Geometry check sheet. Reference: drawing and pictorial views, mm from the part's lowest x, y, z. A direction names the side the tool comes from. Round coordinates to 2 decimals unless told otherwise and drop trailing zeros. Order: outer loops, then holes, each group sorted by start corner. A loop starts at its lowest first (then second) coordinate and runs counter-clockwise, first axis right, second up. Notation, with made-up numbers: (86.25, 89.5) -> (131.25, 89.5) arc R23 cw to (131.25, 128.5) -> close; hole circle Ø10 at (26, 4.25). An arc over 180 degrees is marked (long way). Return JSON: item names as keys, results as strings. Group by question number.
1) Section check D-D on x = 63. Enter the section's corners in (y, z) (1 decimal), plus the area to 3 significant figures.
2) Section check A-A on z = 13. Enter the section's corners in (x, y) (1 decimal), plus the area to 3 significant figures.
3) Section check B-B on y = 1.5. Enter the section's corners in (x, z) (1 decimal).
4) Tool access check on the marked faces 1, 2 and 3. Record the directions out of +Z, -Z, +X, -X, +Y, -Y that give a thin tool (end or side, any length) a straight path to the whole face; none if there is none.
5) Section check C-C on z = 1.5. Enter the section's corners in (x, y) (1 decimal), plus the area to 3 significant figures.
6) Depth check by flat-ended pin: pin 1 (10 mm diameter, centred on x = 67, z = 17, fed in from -Y); pin 2 (2.5 mm diameter, centred on x = 79, y = 2.5, fed in from +Z); pin 3 (2 mm diameter, centred on x = 49.5, z = 3, fed in from +Y); pin 4 (0.8 mm diameter, centred on x = 30, y = 4, fed in from +Z). Enter the tip coordinate at first touch or a pass-through.
7) Scan lines: L1, parallel to X at y = 1, z = 6 (1 decimal); L2, parallel to Y at x = 51.5, z = 1; L3, parallel to X at y = 7.5, z = 17.75. Record each from-to range of solid material in increasing order.
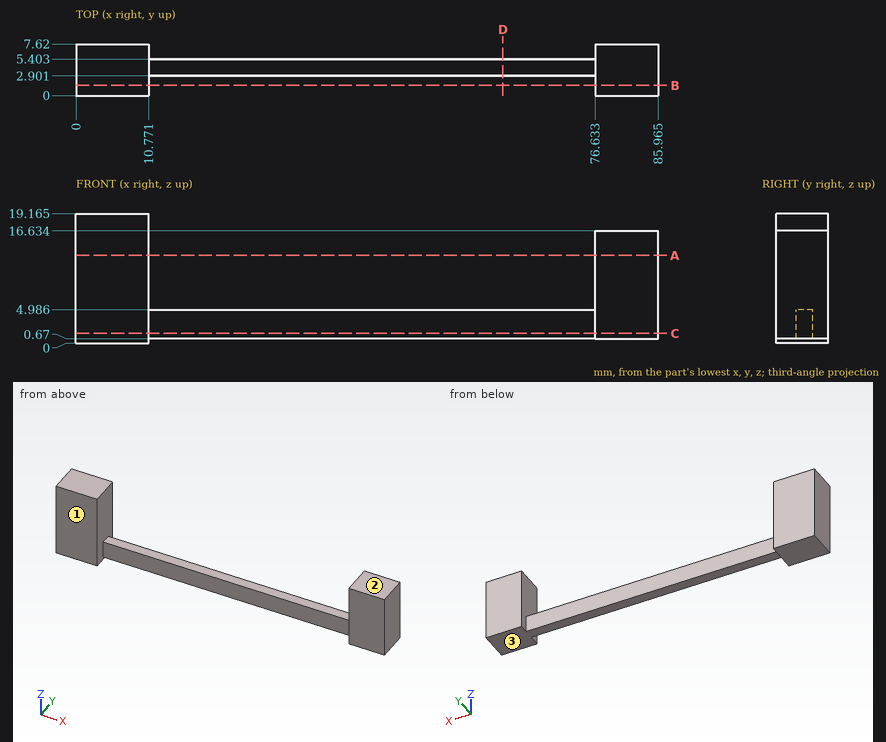
Check result:
{
 "1": {"outline": "(2.9, 0.7) -> (5.4, 0.7) -> (5.4, 5) -> (2.9, 5) -> close", "area": "10.8 mm^2"},
 "2": {"outline": "(0, 0) -> (10.8, 0) -> (10.8, 7.6) -> (0, 7.6) -> close; (76.6, 0) -> (86, 0) -> (86, 7.6) -> (76.6, 7.6) -> close", "area": "153 mm^2"},
 "3": {"outline": "(0, 0) -> (10.8, 0) -> (10.8, 19.2) -> (0, 19.2) -> close; (76.6, 0.7) -> (86, 0.7) -> (86, 16.6) -> (76.6, 16.6) -> close"},
 "4": {"face 1": "+Z, -Z, +X, -X, -Y", "face 2": "+Z, +X, +Y, -Y", "face 3": "-Z, +X, +Y, -Y"},
 "5": {"outline": "(0, 0) -> (10.8, 0) -> (10.8, 2.9) -> (76.6, 2.9) -> (76.6, 0) -> (86, 0) -> (86, 7.6) -> (76.6, 7.6) -> (76.6, 5.4) -> (10.8, 5.4) -> (10.8, 7.6) -> (0, 7.6) -> close", "area": "318 mm^2"},
 "6": {"pin 1": "through", "pin 2": "z = 16.63", "pin 3": "y = 5.4", "pin 4": "z = 4.99"},
 "7": {"L1": "0 to 10.8, 76.6 to 86", "L2": "2.9 to 5.4", "L3": "0 to 10.77"}
}
